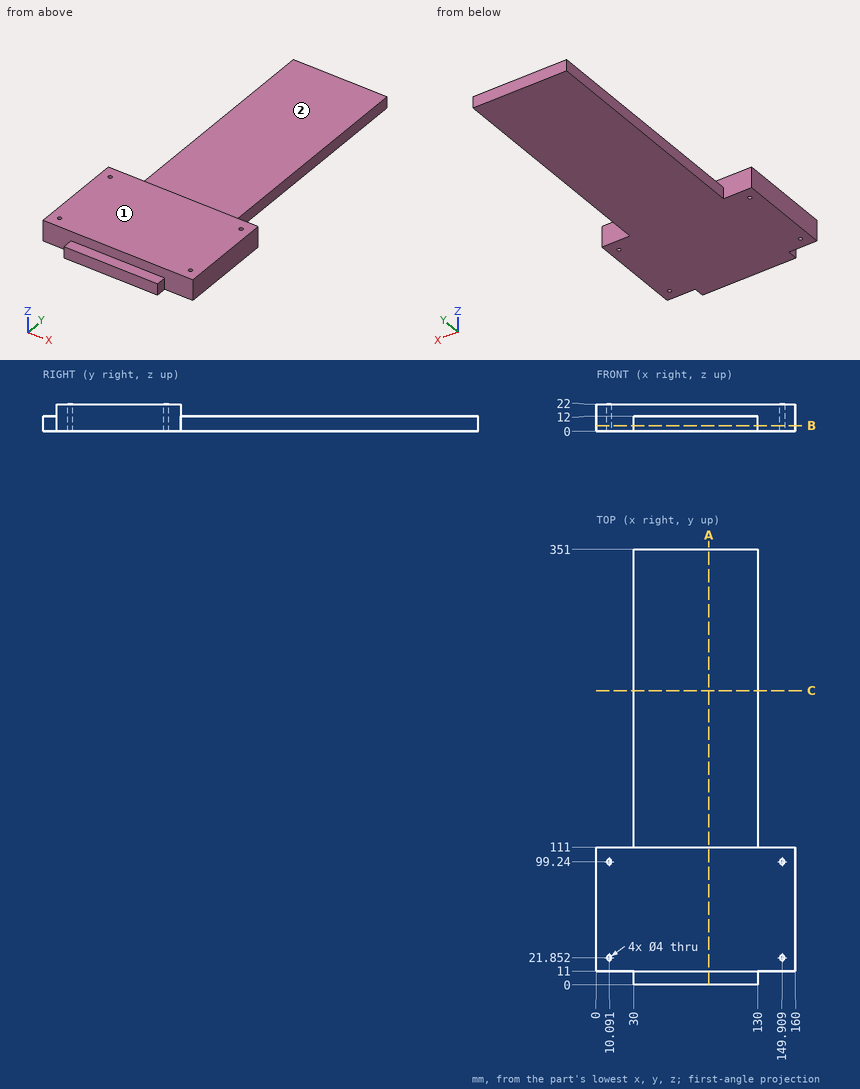
Part print with two shaded views. Sizes in mm from the minimum x, y, z corner. A direction names the side the tool comes from. Round coordinates to 2 decimals unless told otherwise and drop trailing zeros. Loops run counter-clockwise (first coordinate to the right, second up) from the corner with the lowest first, then second, coordinate; pieces in that order, holes last. Notation, with made-up numbers: (-15, -31) - (19, -31) arc R24 cw to (19, 7) - close; hole circle Ø11 at (50, 65.25). An arc over 180 degrees is marked (long way). Put each result on its own line as item: value.
1. Slice it at C-C on y = 237. List the corners of the cut face in (x, z).
Geometry check:
outline: (30, 0) - (130, 0) - (130, 12) - (30, 12) - close
2. 3-axis set-ups, long thin cutter, end or side, ignore diameter. For the marked faces 1 and 2: which of +Z, -Z, +X, -X, +Y, -Y reach the whole face in a straight line?
Geometry check:
face 1: +Z, +X, -X, +Y, -Y
face 2: +Z, +X, -X, +Y
3. Slice it at B-B on z = 4.5. List the corners of the cut face in (x, y).
Geometry check:
outline: (0, 11) - (30, 11) - (30, 0) - (130, 0) - (130, 11) - (160, 11) - (160, 111) - (130, 111) - (130, 351) - (30, 351) - (30, 111) - (0, 111) - close; hole circle Ø4 at (10.09, 21.85); hole circle Ø4 at (10.09, 99.24); hole circle Ø4 at (149.91, 21.85); hole circle Ø4 at (149.91, 99.24)
4. Slice it at A-A on x = 90.5. List the corners of the cut face in (y, z), and give its area (3 significant figures).
Geometry check:
outline: (0, 0) - (351, 0) - (351, 12) - (111, 12) - (111, 22) - (11, 22) - (11, 12) - (0, 12) - close
area: 5,210 mm²
5. Wall check: line 1 (Y direction, x = 16, z = 3.75); line 2 (Z direction, x = 89.5, y = 289); line 3 (X direction, y = 297.5, z = 4.25). Give the ranges that are in metal, low to high.
Geometry check:
line 1: 11 to 111
line 2: 0 to 12
line 3: 30 to 130
6. Pin check, flat tips, straight feed: P1, Ø3.5, axis at x = 64, y = 6.5, coming from the +Z side; P2, Ø5, axis at y = 245, z = 4.5, coming from the -X side; P3, Ø13, axis at y = 273, z = 5, coming from the +X side. Stop position of each tip, or through.
Geometry check:
P1: z = 12
P2: x = 30
P3: x = 130
